```python
from build123d import *

# Parameters (mm, degrees)
F1_DEPTH = 25
F3_DEPTH = 25


with BuildPart() as f1:
    # F0 (on Right) → F1 (new body)
    with BuildSketch(Plane.YZ):
        Polygon((30, 0), (0, 0), (0, -20), (60, -20), align=None)
    extrude(amount=F1_DEPTH)

    # F2 (on face) → F3 (cut)
    with BuildSketch(Plane.YZ.offset(25)):
        with BuildLine():
            Line((30, -20), (0, -20))
            Line((0, -20), (0, -28))
            Line((0, -28), (72, -28))
            Line((72, -28), (53.764115, -15.842743))
            ThreePointArc((53.764115, -15.842743), (42.062503, -18.952854), (30, -20))
        make_face()
    extrude(amount=-F3_DEPTH, mode=Mode.SUBTRACT)


solid = f1.part
```
Design review of the part built by this model. Coordinates are the model's own, in mm. Give positions to 0.01 mm unless a question says otherwise; leave off trailing zeros. Write each loop counter-clockwise with the first axis right and the second up, starting at its lowest first coordinate (ties: lowest second). Pieces come first, ordered by that corner, then holes.
(1) Wall thickness on line 1 along Z through (x, y) = (9, 34.5); line 2 along Y through (x, z) = (23.5, -11.5); line 3 along Z through (x, y) = (21.5, 41): over which ranges is each line inside the solid? List them lowest first.
Checked values:
line 1: z = -19.86 to -3
line 2: y = 0 to 47.25
line 3: z = -19.13 to -7.33
(2) Add section C-C (y = 50.5). Give the boundary of the cut face in (x, z), and give its area (3 significant figures).
Checked values:
outline: (0, -16.93) - (25, -16.93) - (25, -13.67) - (0, -13.67) - close
area: 81.6 mm2
(3) Add section A-A (z = -11). Give the boundary of the cut face in (x, y), and give its area (3 significant figures).
Checked values:
outline: (0, 0) - (25, 0) - (25, 46.5) - (0, 46.5) - close
area: 1,160 mm2
(4) Clearance check with flat-ended pins moving along their axes: pin 1 Ø4 at (x, z) = (4.5, -4.5) entering from +Y; pin 2 Ø2 at (x, y) = (3.5, 40) entering from +Z; pin 3 Ø1.5 at (x, y) = (16, 47.5) entering from -Z. State where each tip first meets the part, or that it passes through.
Checked values:
pin 1: stops at y = 39.75
pin 2: stops at z = -6
pin 3: stops at z = -17.97
(5) Add section B-B (x = 15.25). Give the boundary of the cut face in (y, z), and give its area (3 significant figures).
Checked values:
outline: (0, -20) - (30, -20) arc R70 ccw to (53.76, -15.84) - (30, 0) - (0, 0) - close
area: 855 mm2
(6) Mouldability with a two-part tool opening along X and no side actions: class faces 1 (the face through (25, 21, -10)), 2 (the face through (0, 21, -10)), 3 (the face through (12, 0, -10)) as +X half, -X half, draft (parallel to the pull), parting line (faces both ways), or undercut.
Checked values:
face 1: +X half
face 2: -X half
face 3: draft
